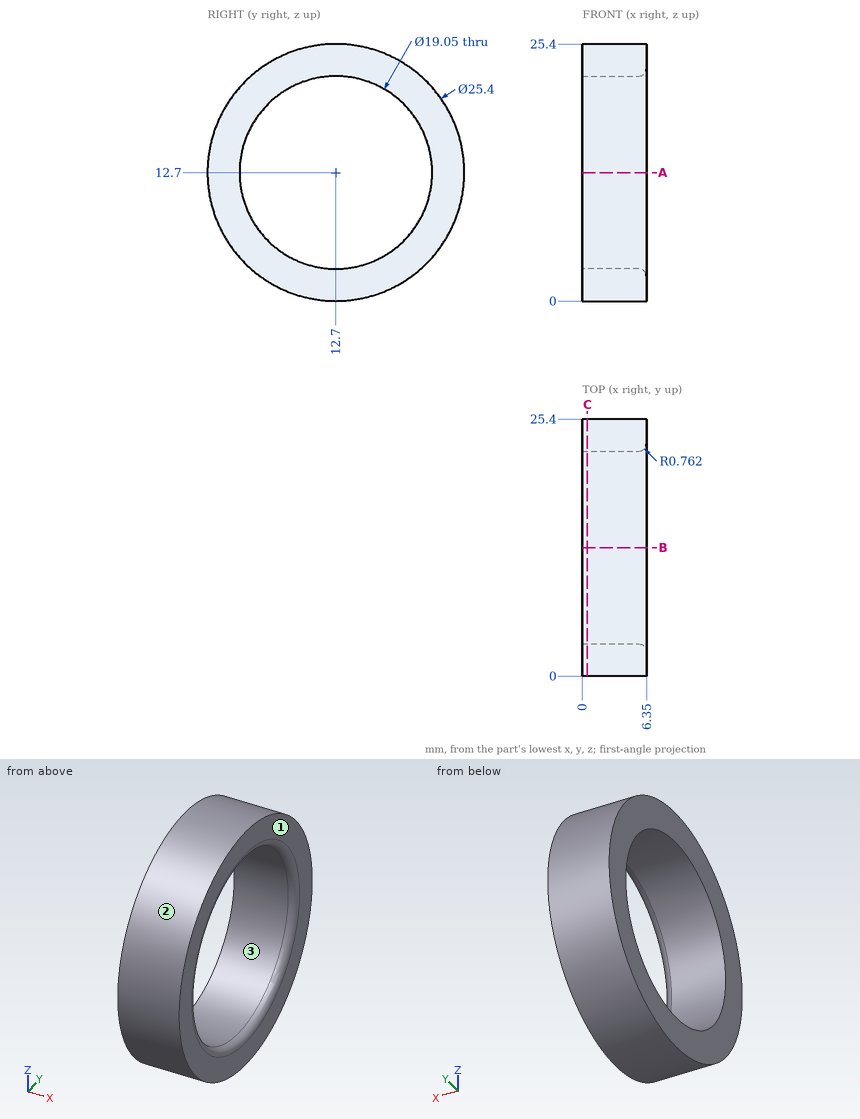
Study the drawing (mm; zero at the part's minimum x, y, z) and answer. Round coordinates to 2 decimals unless told otherwise and drop trailing zeros. Write each loop counter-clockwise with the first axis right and the second up, starting at its lowest first coordinate (ties: lowest second). Pieces come first, ordered by that corner, then holes. Notation, with made-up numbers: (-29.75, -40) - (-1.75, -40) arc R16 ccw to (-1.75, -36) - close; hole circle Ø1 at (3.25, 3.5). An arc over 180 degrees is marked (long way). Use a Markdown table: item, result. Add a question column.
1. The part is cut by section A-A (z = 12.7). Write down the section's boundary in (x, y) (3 decimals), and give its area (3 significant figures).
2. Consider line 1 (Y direction, x = 3.45, z = 12.7) (3 decimals); line 2 (Z direction, x = 4, y = 13); line 3 (Z direction, x = 2.75, y = 18.5). Determine where each line is inside the solid, lowest interval first.
3. For a pull along Z with two mould halves and no side action, classify the marked faces 1, 2 and 3 as +Z half, -Z half, draft (parallel to the pull), parting line (faces both ways), or undercut.
4. The part is cut by section C-C (x = 0.5). Write down the section's boundary in (y, z) (3 decimals), and give its area (3 significant figures).
5. Flat-ended cylindrical pins translate along their axes: P1, Ø3, axis at x = 1.5, z = 5.5, coming from the +Y side; P2, Ø1, axis at x = 3.5, z = 11.5, coming from the +Y side; P3, Ø1, axis at x = 3.5, z = 9.5, coming from the +Y side. Find the tip coordinate at first contact, or state that the pin passes through.
Reported:
| question | item | result |
|---|---|---|
| 1 | outline | (0, 0) - (6.35, 0) - (6.35, 2.413) arc R0.762 ccw to (5.588, 3.175) - (0, 3.175) - close; (0, 22.225) - (5.588, 22.225) arc R0.762 ccw to (6.35, 22.987) - (6.35, 25.4) - (0, 25.4) - close |
| 1 | area | 40.1 mm^2 |
| 2 | line 1 | 0 to 3.175, 22.225 to 25.4 |
| 2 | line 2 | 0 to 3.18, 22.22 to 25.4 |
| 2 | line 3 | 1.4 to 5.14, 20.26 to 24 |
| 3 | face 1 | draft |
| 3 | face 2 | parting line |
| 3 | face 3 | undercut |
| 4 | outline | circle Ø25.4 at (12.7, 12.7); hole circle Ø19.05 at (12.7, 12.7) |
| 4 | area | 222 mm^2 |
| 5 | P1 | y = 24.05 |
| 5 | P2 | y = 25.38 |
| 5 | P3 | y = 25.11 |
